```python
from build123d import *

# Parameters (mm, degrees)
F0_R      = 12.7
F1_DEPTH  = 60.325
F2_DEPTH  = 41.275
F0_W      = 32.8422
F0_H      = 22.352
F4_DEPTH  = 41.275
F5_DEPTH  = 19.05
F0_W_2    = 44.1198
F6_DEPTH  = 41.275
F7_DEPTH  = 19.05
F8_W      = 22.3266
F8_H      = 44.704
F9_DEPTH  = 47.752
F10_R     = 6.35
F11_DEPTH = 22.352
F12_R     = 5.08
F13_R     = 7.874
F14_W     = 22.2758
F14_H     = 4.605526296
F15_DEPTH = 22.352


with BuildPart() as f1:
    # F0 (on Right) → F1 (new body)
    with BuildSketch(Plane.YZ):
        with BuildLine():
            ThreePointArc((-94.8944, 22.352), (-133.0516507731, 38.1572507731), (-117.2464, 0))
            Line((-117.2464, 0), (-25.4, 0))
            Line((-25.4, 0), (-31.3944, 22.352))
            Line((-31.3944, 22.352), (-94.8944, 22.352))
        make_face()
        with Locations((-117.2464, 22.352)):
            Circle(F0_R, mode=Mode.SUBTRACT)
    extrude(amount=-F1_DEPTH)

    # F0 (on Right) → F2 (join)
    with BuildSketch(Plane.YZ):
        Polygon((-31.3944, 22.352), (-25.4, 0), (0, 0), (0, 22.352), align=None)
    extrude(amount=-F2_DEPTH)


with BuildPart() as f1_1:
    # F3: moved
    add(f1.part.moved(Location((41.275, 0, 0))))

    # F0 (on Right) → F4 (join)
    with BuildSketch(Plane.YZ):
        with Locations((16.4211, 11.176)):
            Rectangle(F0_W, F0_H)
    extrude(amount=F4_DEPTH)

    # F0 (on Right) → F5 (join)
    with BuildSketch(Plane.YZ):
        with Locations((16.4211, 11.176)):
            Rectangle(F0_W, F0_H)
        with BuildLine():
            ThreePointArc((13.7922, 57.15), (10.2180153616, 38.4343576341), (0, 22.352))
            Line((0, 22.352), (32.8422, 22.352))
            Line((32.8422, 22.352), (32.8422, 57.15))
            Line((32.8422, 57.15), (13.7922, 57.15))
        make_face()
    extrude(amount=-F5_DEPTH)

    # F0 (on Right) → F6 (join)
    with BuildSketch(Plane.YZ):
        with Locations((54.9021, 11.176)):
            Rectangle(F0_W_2, F0_H)
    extrude(amount=F6_DEPTH)

    # F0 (on Right) → F7 (join)
    with BuildSketch(Plane.YZ):
        with Locations((54.9021, 11.176)):
            Rectangle(F0_W_2, F0_H)
    extrude(amount=-F7_DEPTH)

    # F8 (on Top) → F9 (cut)
    with BuildSketch(Plane.XY):
        with Locations((11.1125, -117.2464)):
            Rectangle(F8_W, F8_H)
    extrude(amount=F9_DEPTH, mode=Mode.SUBTRACT)

    # F10 (on face) → F11 (cut)
    with BuildSketch(Plane.XY.offset(22.352)):
        with Locations((18.923, 38.1)):
            Circle(F10_R)
    extrude(amount=-F11_DEPTH, mode=Mode.SUBTRACT)

    # F12
    f12_edges = [f1_1.edges().sort_by_distance(p)[0] for p in [
        (-9.525, 32.8422, 57.15),
        (-9.525, 32.8422, 22.352),
        (-9.5504, -94.8944, 22.352),
        (31.7754, -94.8944, 22.352),
    ]]
    fillet(f12_edges, radius=F12_R)

    # F13
    f13_edges = [f1_1.edges().sort_by_distance(p)[0] for p in [
        (11.1125, 76.962, 22.352),
    ]]
    fillet(f13_edges, radius=F13_R)

    # F14 (on face) → F15 (cut)
    with BuildSketch(Plane.XY.offset(22.352)):
        with Locations((11.1379, -92.591636852)):
            Rectangle(F14_W, F14_H)
    extrude(amount=-F15_DEPTH, mode=Mode.SUBTRACT)


solid = f1_1.part
```
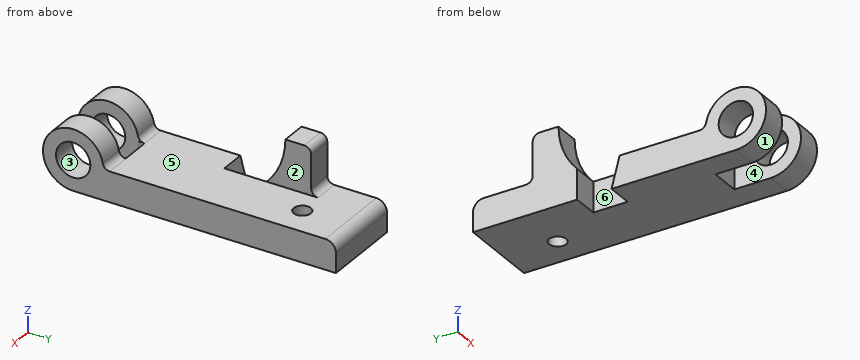
The listing builds one solid part. Answer for the finished solid, in the listing's coordinates (mm). Face numbers are marked on the shaded views. A direction names the side the tool comes from. Coordinates: 2 decimals unless noted, no trailing zeros. Loops run counter-clockwise (first coordinate to the right, second up) from the corner with the lowest first, then second, coordinate; pieces in that order, holes last. Notation, with made-up numbers: (-2, -28.5) -> (5, -28.5) arc R22 ccw to (5, -11.5) -> close; hole circle Ø8 at (6, -33). An arc over 180 degrees is marked (long way). Return JSON: item names as keys, results as strings. Group by question number.
(1) A cutting plane is placed at D-D on x = 35. Write down the section's boundary in (y, z).
(2) A cutting plane is placed at A-A on x = -2. Write down the section's boundary in (y, z), and give its area (3 significant figures).
(3) Given pin 1 Ø15 at (x, z) = (-5, 36) entering from +Y; pin 2 Ø5.5 at (x, z) = (-9, 14.5) entering from -Y; pin 3 Ø24.5 at (x, z) = (6.5, 11) entering from -Y, each flat-ended and moving along its own axis, determine where each tip first touches the part or whether it passes through.
(4) Determine the mould class of the marked faces 1, 2 and 3 for opening direction Z: released by +Z, released by -Z, zero draft, split by the parting line, or undercut.
(5) A cutting plane is placed at C-C on x = 20. Write down the section's boundary in (y, z), and give its area (3 significant figures).
(6) Which of the six approach directions +Z, -Z, +X, -X, +Y, -Y give full straight-line access (tool end or side, diameter ignored) to the marked faces 4, 5 and 6?
(7) A cutting plane is placed at B-B on z = 42. Write down the section's boundary in (x, y) (3 decimals).
(8) Find the intervals of material crossed by probe 1 along Z at (x, y) = (-4.5, -118); probe 2 along X at (y, z) = (-95, 3) (3 decimals); probe 3 along Z at (x, y) = (7.5, 17.5), in increasing order. Write a range as from..to.
The answers:
{
 "1": {"outline": "(-117.25, 0) -> (76.96, 0) -> (76.96, 14.48) arc R7.87 ccw to (69.09, 22.35) -> (-90.29, 22.35) arc R5.08 cw to (-95.28, 26.49) arc R22.35 ccw (long way) to start; hole circle Ø25.4 at (-117.25, 22.35)"},
 "2": {"outline": "(-117.25, 0) -> (-25.4, 0) -> (-31.39, 22.35) -> (-90.29, 22.35) arc R5.08 cw to (-95.28, 26.49) arc R22.35 ccw (long way) to start; (0, 0) -> (76.96, 0) -> (76.96, 14.48) arc R7.87 ccw to (69.09, 22.35) -> (37.92, 22.35) arc R5.08 cw to (32.84, 27.43) -> (32.84, 52.07) arc R5.08 ccw to (27.76, 57.15) -> (13.79, 57.15) arc R50.8 cw to (0, 22.35) -> close; hole circle Ø25.4 at (-117.25, 22.35)", "area": "5,180 mm^2"},
 "3": {"pin 1": "stops at y = 32.84", "pin 2": "stops at y = -139.01", "pin 3": "stops at y = -139.58"},
 "4": {"face 1": "split by the parting line", "face 2": "zero draft", "face 3": "undercut"},
 "5": {"outline": "(-90.29, 0) -> (31.84, 0) -> (31.84, 22.35) -> (-90.29, 22.35) -> close; (44.36, 0) -> (76.96, 0) -> (76.96, 14.48) arc R7.87 ccw to (69.09, 22.35) -> (44.36, 22.35) -> close", "area": "3,450 mm^2"},
 "6": {"face 4": "+Z, -Z, -Y", "face 5": "+Z, +X", "face 6": "+Z, -X"},
 "7": {"outline": "(-19.05, -127.903) -> (-0.051, -127.903) -> (-0.051, -106.59) -> (-19.05, -106.59) -> close; (-19.05, 11.48) -> (0, 11.48) -> (0, 32.842) -> (-19.05, 32.842) -> close; (22.276, -127.903) -> (41.275, -127.903) -> (41.275, -106.59) -> (22.276, -106.59) -> close"},
 "8": {"probe 1": "z = 0.01..9.67, 35.03..44.69", "probe 2": "x = -19.05..-0.051, 22.276..41.275", "probe 3": "z = 0..22.35"}
}
